Read the model definition and answer for the solid it produces. Units are mm, in the model's axes. Face numbers are marked on the shaded views. A direction names the side the tool comes from. Give positions to 0.01 mm unless a question says otherwise; leave off trailing zeros. Write each loop counter-clockwise with the first axis right and the second up, starting at its lowest first coordinate (ties: lowest second). Pieces come first, ordered by that corner, then holes. Notation, with made-up numbers: (57.25, 24.5) -> (112.25, 24.5) arc R15 ccw to (112.25, 46.5) -> close; hole circle Ø8 at (-15.75, -2). An arc over 180 degrees is marked (long way). Use a Markdown table: item, result.
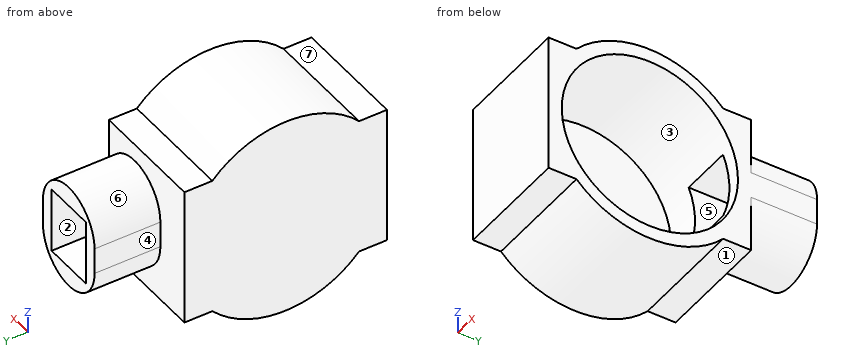
from build123d import *

# Parameters (mm, degrees)
SKETCH1_R                = 38.45
BOSS_EXTRUDE1_DEPTH      = 55.5
SHELL1_T                 = -5
BOSS_EXTRUDE2_REACH      = 104.334
BOSS_EXTRUDE2_END_RADIUS = 38.45
SKETCH2_W                = 111
SKETCH2_H                = 53.04
CUT_EXTRUDE1_REACH       = 104.334
CUT_EXTRUDE1_END_RADIUS  = 33.45
SKETCH3_W                = 20
SKETCH3_H                = 25
BOSS_EXTRUDE5_DEPTH      = 25
CUT_EXTRUDE2_REACH       = 124.239
SKETCH6_W                = 20
SKETCH6_H                = 25
CUT_EXTRUDE3_DEPTH       = 103.334073016
CUT_EXTRUDE3_DEPTH_BACK  = 103.334073016
SKETCH7_W                = 67
SKETCH7_H                = 76.9


with BuildPart() as part:
    # Sketch1 → Boss-Extrude1 (new, symmetric)
    with BuildSketch(Plane(origin=(0, 0, 0), x_dir=(0, 0, -1), z_dir=(1, 0, 0))):
        Circle(SKETCH1_R)
    extrude(amount=BOSS_EXTRUDE1_DEPTH, both=True)

    # Shell1
    shell1_openings = [part.faces().sort_by_distance(p)[0] for p in [
        (55.5, 0, 0),
    ]]
    offset(amount=SHELL1_T, openings=shell1_openings, kind=Kind.INTERSECTION)

    # Boss-Extrude2: up to this cylinder (the profile starts outside it)
    boss_extrude2_end = Plane(origin=(0, 0, 0), z_dir=(-1, 0, 0)) * Cylinder(BOSS_EXTRUDE2_END_RADIUS, 286.568, mode=Mode.PRIVATE)
    # Sketch2 → Boss-Extrude2 (add, up to the surface)
    with BuildSketch(Plane(origin=(0, 38.45, 0), x_dir=(1, 0, 0), z_dir=(0, 1, 0)), mode=Mode.PRIVATE) as boss_extrude2_sk1:
        Rectangle(SKETCH2_W, SKETCH2_H)
    boss_extrude2_tool1 = extrude(boss_extrude2_sk1.sketch, amount=-BOSS_EXTRUDE2_REACH, mode=Mode.PRIVATE) - boss_extrude2_end
    boss_extrude2 = boss_extrude2_tool1.solids().sort_by_distance((0, 38.45, 0))[0] + boss_extrude2_tool1.solids().sort_by_distance((0, 38.45, 0))[1]
    add(boss_extrude2)

    # Mirror1: Boss-Extrude2 across plane
    add(boss_extrude2.mirror(Plane.ZX))

    # Cut-Extrude1: up to this cylinder (the profile starts outside it)
    cut_extrude1_end = Plane(origin=(-26.5, 0, 0), z_dir=(-1, 0, 0)) * Cylinder(CUT_EXTRUDE1_END_RADIUS, 276.568, mode=Mode.PRIVATE)
    # Sketch3 → Cut-Extrude1 (cut, up to the surface)
    with BuildSketch(Plane(origin=(0, 38.45, 0), x_dir=(1, 0, 0), z_dir=(0, 1, 0)), mode=Mode.PRIVATE) as cut_extrude1_sk1:
        with Locations((-26.5, 0)):
            Rectangle(SKETCH3_W, SKETCH3_H)
    cut_extrude1_tool1 = extrude(cut_extrude1_sk1.sketch, amount=-CUT_EXTRUDE1_REACH, mode=Mode.PRIVATE) - cut_extrude1_end
    add(cut_extrude1_tool1.solids().sort_by_distance((-26.5, 38.45, 0))[0], mode=Mode.SUBTRACT)

    # Sketch5 → Boss-Extrude5 (add)
    with BuildSketch(Plane(origin=(0, 38.45, 0), x_dir=(1, 0, 0), z_dir=(0, 1, 0))):
        with BuildLine():
            Line((-11.5, 5), (-11.5, -5))
            ThreePointArc((-11.5, -5), (-26.5, -20), (-41.5, -5))
            Line((-41.5, -5), (-41.5, 5))
            ThreePointArc((-41.5, 5), (-26.5, 20), (-11.5, 5))
        make_face()
    extrude(amount=BOSS_EXTRUDE5_DEPTH)

    # Sketch6 → Cut-Extrude2 (cut, up to next)
    with BuildSketch(Plane(origin=(0, 63.45, 0), x_dir=(1, 0, 0), z_dir=(0, 1, 0)), mode=Mode.PRIVATE) as cut_extrude2_sk1:
        with Locations((-26.5, 0)):
            Rectangle(SKETCH6_W, SKETCH6_H)
    cut_extrude2_tool1 = extrude(cut_extrude2_sk1.sketch, amount=-CUT_EXTRUDE2_REACH, mode=Mode.PRIVATE) & part.part
    add(cut_extrude2_tool1.solids().sort_by_distance((-26.5, 63.45, 0))[0], mode=Mode.SUBTRACT)

    # Sketch7 → Cut-Extrude3 (cut, two sides: drawn at the far end of the back side and taken through both)
    with BuildSketch(Plane(origin=(0, 38.45, 0), x_dir=(1, 0, 0), z_dir=(0, 1, 0)).offset(-CUT_EXTRUDE3_DEPTH_BACK)):
        with Locations((22, 0)):
            Rectangle(SKETCH7_W, SKETCH7_H)
    extrude(amount=CUT_EXTRUDE3_DEPTH + CUT_EXTRUDE3_DEPTH_BACK, mode=Mode.SUBTRACT)


solid = part.part
Item 1: A cutting plane is placed at A-A (z = 0). Give the vertices of the cut face in (x, y).
Return value:
| item | result |
|---|---|
| outline | (-55.5, -38.45) -> (-11.5, -38.45) -> (-11.5, -33.45) -> (-50.5, -33.45) -> (-50.5, 33.45) -> (-36.5, 33.45) -> (-36.5, 63.45) -> (-41.5, 63.45) -> (-41.5, 38.45) -> (-55.5, 38.45) -> close; (-16.5, 33.45) -> (-11.5, 33.45) -> (-11.5, 63.45) -> (-16.5, 63.45) -> close |
Item 2: A cutting plane is placed at C-C (y = 0). Give the vertices of the cut face in (x, z), then the cut area to 4 significant figures.
Return value:
| item | result |
|---|---|
| outline | (-55.5, -38.45) -> (-11.5, -38.45) -> (-11.5, -33.45) -> (-50.5, -33.45) -> (-50.5, 33.45) -> (-11.5, 33.45) -> (-11.5, 38.45) -> (-55.5, 38.45) -> close |
| area | 774.5 mm^2 |
Item 3: A cutting plane is placed at D-D (x = -26.5). Give the vertices of the cut face in (y, z), then the cut area to 3 significant figures.
Return value:
| item | result |
|---|---|
| outline | (-38.45, -26.52) -> (-27.84, -26.52) arc R38.45 ccw to (27.84, -26.52) -> (38.45, -26.52) -> (38.45, -20) -> (63.45, -20) -> (63.45, -12.5) -> (31.03, -12.5) arc R33.45 cw (long way) to (31.03, 12.5) -> (63.45, 12.5) -> (63.45, 20) -> (38.45, 20) -> (38.45, 26.52) -> (27.84, 26.52) arc R38.45 ccw to (-27.84, 26.52) -> (-38.45, 26.52) -> close |
| area | 1,710 mm^2 |
Item 4: Straight lines are drawn through the part: line 1 along Y through (x, z) = (-40, 0); line 2 along X through (y, z) = (36.5, 11); line 3 along Z through (x, y) = (-31.5, 25.5). For each, find the intervals that lie inside material, in ascending order. Write a range as [from, to].
Return value:
| item | result |
|---|---|
| line 1 | [-38.45, -33.45], [33.45, 63.45] |
| line 2 | [-55.5, -36.5], [-16.5, -11.5] |
| line 3 | [-28.78, -21.65], [21.65, 28.78] |
Item 5: A tool of negligible diameter and unlimited length cuts with its end or side. For the marked faces 1, 2, 3 and 4, from which of +Z, -Z, +X, -X, +Y, -Y can it reach the whole face along a straight path? Write none if from no direction.
Return value:
| item | result |
|---|---|
| face 1 | -Z, +X, -X, +Y |
| face 2 | +Y |
| face 3 | +X |
| face 4 | +Z, -Z, -X, +Y |
Item 6: For a pull along X with two mould halves and no side action, classify the marked faces 5, 6 and 7 as +X half, -X half, draft (parallel to the pull), parting line (faces both ways), or undercut.
Return value:
| item | result |
|---|---|
| face 5 | undercut |
| face 6 | parting line |
| face 7 | draft |
Item 7: Each of these flat-tipped pins is pushed along its axis until it touches: P1, Ø5, axis at y = 3, z = -5.5, coming from the +X side; P2, Ø3, axis at y = 49.5, z = -2.5, coming from the -X side; P3, Ø10, axis at x = -46, y = -4, coming from the +Z side; P4, Ø10, axis at x = -21.5, y = 53.5, coming from the -Z side. Where does it stop, or does it pass through?
Return value:
| item | result |
|---|---|
| P1 | x = -50.5 |
| P2 | x = -41.5 |
| P3 | z = 38.45 |
| P4 | z = -20 |
Item 8: A cutting plane is placed at B-B (x = -47). Give the vertices of the cut face in (y, z), then the cut area to 3 significant figures.
Return value:
| item | result |
|---|---|
| outline | (-38.45, -26.52) -> (-27.84, -26.52) arc R38.45 ccw to (27.84, -26.52) -> (38.45, -26.52) -> (38.45, 26.52) -> (27.84, 26.52) arc R38.45 ccw to (-27.84, 26.52) -> (-38.45, 26.52) -> close; hole circle Ø66.9 at (0, 0) |
| area | 1,480 mm^2 |
